CAD build for the part. Positions are in the model's coordinates, mm. Face numbers are marked on the shaded views. A direction names the side the tool comes from. Round coordinates to 2 decimals unless told otherwise and drop trailing zeros. Order: outer loops, then holes, each group sorted by start corner. A loop starts at its lowest first (then second) coordinate and runs counter-clockwise, first axis right, second up. Notation, with made-up numbers: M 61.25,63.5 L 92.25,63.5 A15 ccw 92.25,88.5 Z; hole C 86.25,44 d2. An arc over 180 degrees is marked long. Answer as CSV lines item,"result". Start each with the question number.
```python
from build123d import *

# Parameters (mm, degrees)
SKICA1_W                = 300
SKICA1_H                = 300
P_IDAT_VYSUNUT_M1_DEPTH = 10
P_IDAT_VYSUNUT_M3_DEPTH = 10


with BuildPart() as part:
    # Skica1 → Přidat vysunutím1 (new body)
    with BuildSketch(Plane.XY):
        with Locations((150, 150)):
            Rectangle(SKICA1_W, SKICA1_H)
    extrude(amount=P_IDAT_VYSUNUT_M1_DEPTH)

    # Skica3 → Přidat vysunutím3 (add)
    with BuildSketch(Plane.XY.offset(10)):
        with BuildLine():
            Line((153.157459628, 57.904394304), (138.29070055, 56.980883154))
            ThreePointArc((138.29070055, 56.980883154), (110.247943411, 65.348513102), (94.289058074, 89.878646361))
            ThreePointArc((94.289058074, 89.878646361), (103.547245504, 146.603196293), (149.788099838, 180.737812008))
            ThreePointArc((149.788099838, 180.737812008), (154.882621426, 181.830553973), (160.045482007, 182.53276892))
            ThreePointArc((160.045482007, 182.53276892), (168.864101161, 178.213116415), (168.96323198, 168.393869264))
            ThreePointArc((168.96323198, 168.393869264), (161.268139192, 156.982073578), (152.456108269, 146.408916775))
            ThreePointArc((152.456108269, 146.408916775), (132.164950971, 127.005263014), (109.623212842, 110.268988463))
            ThreePointArc((109.623212842, 110.268988463), (102.928809573, 102.150565652), (102.087824963, 91.661687307))
            ThreePointArc((102.087824963, 91.661687307), (115.038295459, 71.755737716), (137.794703021, 64.965492503))
            Line((137.794703021, 64.965492503), (152.6614621, 65.889003653))
            ThreePointArc((152.6614621, 65.889003653), (156.901765538, 62.144697743), (153.157459628, 57.904394304))
        make_face()
        with BuildLine():
            Line((215.157459628, 57.904394304), (200.29070055, 56.980883154))
            ThreePointArc((200.29070055, 56.980883154), (172.247943411, 65.348513102), (156.289058074, 89.878646361))
            ThreePointArc((156.289058074, 89.878646361), (165.547245504, 146.603196293), (211.788099838, 180.737812008))
            ThreePointArc((211.788099838, 180.737812008), (216.882621426, 181.830553973), (222.045482007, 182.53276892))
            ThreePointArc((222.045482007, 182.53276892), (230.864101161, 178.213116415), (230.96323198, 168.393869264))
            ThreePointArc((230.96323198, 168.393869264), (223.268139192, 156.982073578), (214.456108269, 146.408916775))
            ThreePointArc((214.456108269, 146.408916775), (194.164950971, 127.005263014), (171.623212842, 110.268988463))
            ThreePointArc((171.623212842, 110.268988463), (164.928809573, 102.150565652), (164.087824963, 91.661687307))
            ThreePointArc((164.087824963, 91.661687307), (177.038295459, 71.755737716), (199.794703021, 64.965492503))
            Line((199.794703021, 64.965492503), (214.6614621, 65.889003653))
            ThreePointArc((214.6614621, 65.889003653), (218.901765538, 62.144697743), (215.157459628, 57.904394304))
        make_face()
        with BuildLine():
            Line((277.157459628, 57.904394304), (262.29070055, 56.980883154))
            ThreePointArc((262.29070055, 56.980883154), (234.247943411, 65.348513102), (218.289058074, 89.878646361))
            ThreePointArc((218.289058074, 89.878646361), (227.547245504, 146.603196293), (273.788099838, 180.737812008))
            ThreePointArc((273.788099838, 180.737812008), (278.882621426, 181.830553973), (284.045482007, 182.53276892))
            ThreePointArc((284.045482007, 182.53276892), (292.864101161, 178.213116415), (292.96323198, 168.393869264))
            ThreePointArc((292.96323198, 168.393869264), (285.268139192, 156.982073578), (276.456108269, 146.408916775))
            ThreePointArc((276.456108269, 146.408916775), (256.164950971, 127.005263014), (233.623212842, 110.268988463))
            ThreePointArc((233.623212842, 110.268988463), (226.928809573, 102.150565652), (226.087824963, 91.661687307))
            ThreePointArc((226.087824963, 91.661687307), (239.038295459, 71.755737716), (261.794703021, 64.965492503))
            Line((261.794703021, 64.965492503), (276.6614621, 65.889003653))
            ThreePointArc((276.6614621, 65.889003653), (280.901765538, 62.144697743), (277.157459628, 57.904394304))
        make_face()
    extrude(amount=P_IDAT_VYSUNUT_M3_DEPTH)


solid = part.part
```
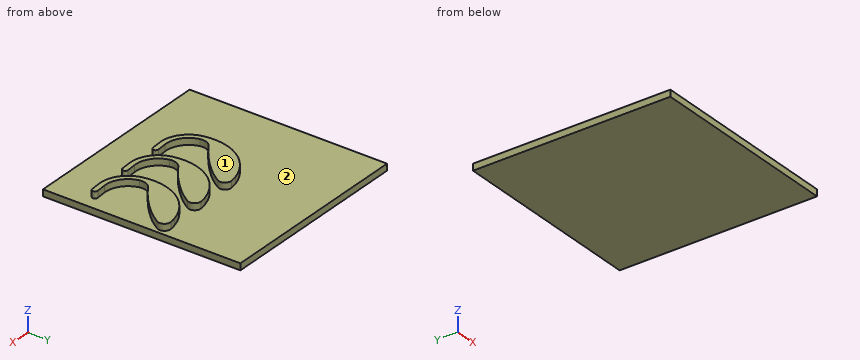
Q1. Band-saw the part on A-A, the plane z = 13.5. Count the separate pieces of the cut face and the enclosed holes in it, then the cut area to 3 significant figures.
Q2. Tool access for the marked faces 1 and 2: list every direction of +Z, -Z, +X, -X, +Y, -Y with a clear straight run to the whole face (end or side of a thin tool).
Q3. Band-saw the part on B-B, the plane x = 204. Write the cut outline in (y, z).
Q4. Probe line 1 along Y through (x, z) = (231.5, 17); line 2 along X through (y, z) = (129.5, 13); line 3 along Z through (x, y) = (106.5, 190). List the from-to ranges inside material, lowest first. Write a range as from..to.
Q5. Drop flat-ended pins along their axis: P1, Ø8, axis at x = 187, y = 200.5, coming from the +Z side; P2, Ø1, axis at y = 134, z = 16, coming from the +X side; P3, Ø12, axis at x = 109.5, z = 17, coming from the +Y side. Give the stop position or say it passes through.
Q6. Band-saw the part on C-C, the plane y = 141. Write the cut outline in (x, z).
Q7. Band-saw the part on D-D, the plane x = 238. Write the cut outline in (y, z).
Answer:
1,separate pieces,"3"
1,enclosed holes,"0"
1,area,"10,900 mm^2"
2,face 1,"+Z, +X, -X, +Y, -Y"
2,face 2,"+Z"
3,outline,"M 0,0 L 300,0 L 300,10 L 178.3,10 L 178.3,20 L 135.81,20 L 135.81,10 L 65.23,10 L 65.23,20 L 57.21,20 L 57.21,10 L 0,10 Z"
4,line 1,"y = 67.59..79.51, 108.65..152.45, 169.42..177.02"
4,line 2,"x = 95.81..135.07, 157.81..197.07, 219.81..259.07"
4,line 3,"z = 0..10"
5,P1,"stops at z = 10"
5,P2,"stops at x = 264.61"
5,P3,"stops at y = 161.56"
6,outline,"M 0,0 L 300,0 L 300,10 L 271.29,10 L 271.29,20 L 224.44,20 L 224.44,10 L 209.29,10 L 209.29,20 L 162.44,20 L 162.44,10 L 147.29,10 L 147.29,20 L 100.44,20 L 100.44,10 L 0,10 Z"
7,outline,"M 0,0 L 300,0 L 300,10 L 160.06,10 L 160.06,20 L 113.19,20 L 113.19,10 L 72.56,10 L 72.56,20 L 62.84,20 L 62.84,10 L 0,10 Z"
